Input: part model. Units: mm. Frame: model coordinates. Give positions to 0.01 mm unless a question says otherwise; leave off trailing zeros. Loops run counter-clockwise (first coordinate to the right, second up) from the corner with the lowest first, then second, coordinate; pieces in that order, holes last. Notation, with made-up numbers: M 75,32 L 115,32 A17 ccw 115,60 Z; hole C 34,80.5 d3. An arc over 180 degrees is marked long. Answer as a JSON object with one key per item and string values. Group by question number.
1) Section query A-A on z = 1. Return loops of the section in (x, y).
2) Section query B-B on x = -102. Return loops of the section in (y, z) (3 decimals), plus the area to 3 significant figures.
3) First-contact query: P1, Ø1.9, axis at y = 2.5, z = 37.5, coming from the -X side; P2, Ø1.9, axis at x = -59, y = 4, coming from the +Z side (3 decimals); P3, Ø1.9, axis at y = 2.5, z = 39.5, coming from the +X side; P4, Ø1.5, axis at x = -86, z = 26.5, coming from the -Y side. Flat tips, straight axial feed; report the tip coordinate or a pass-through.
4) Ray query, L1, parallel to X at y = 4.5, z = 29; L2, parallel to Z at x = 55, y = 1.5 (3 decimals); L3, parallel to X at y = 1.75, z = 1.5. Return the intervals inside material, ascending.
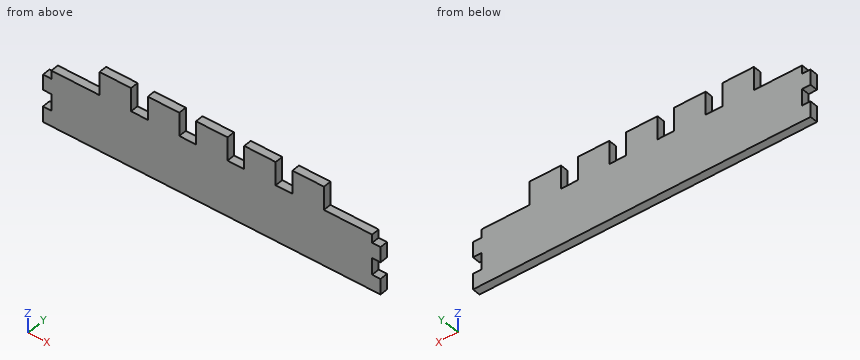
from build123d import *

# Parameters (mm, degrees)
SKETCH1_W           = 266.7
SKETCH1_H           = 57.15
BOSS_EXTRUDE1_DEPTH = 6.35
SKETCH3_W           = 24.892
SKETCH3_H           = 18.542
BOSS_EXTRUDE2_DEPTH = 6.35
SKETCH4_W           = 13.208
SKETCH4_H           = 13.208
CUT_EXTRUDE2_DEPTH  = 142.5717369
SKETCH5_W           = 295.464136086
SKETCH5_H           = 12.7
CUT_EXTRUDE3_DEPTH  = 142.5717369
SKETCH6_W           = 266.7
SKETCH6_H           = 12.446
BOSS_EXTRUDE3_DEPTH = 6.35


with BuildPart() as part:
    # Sketch1 → Boss-Extrude1 (new body)
    with BuildSketch(Plane(origin=(0, 0, 0), x_dir=(1, 0, 0), z_dir=(0, 1, 0))):
        Rectangle(SKETCH1_W, SKETCH1_H)
    extrude(amount=BOSS_EXTRUDE1_DEPTH)

    # Sketch3 → Boss-Extrude2 (add)
    with BuildSketch(Plane(origin=(0, 0, 0), x_dir=(1, 0, 0), z_dir=(0, 1, 0))):
        with Locations((-76.2, -37.846)):
            Rectangle(SKETCH3_W, SKETCH3_H)
        with Locations((-38.1, -37.846)):
            Rectangle(SKETCH3_W, SKETCH3_H)
        with Locations((0, -37.846)):
            Rectangle(SKETCH3_W, SKETCH3_H)
        with Locations((38.1, -37.846)):
            Rectangle(SKETCH3_W, SKETCH3_H)
        with Locations((76.2, -37.846)):
            Rectangle(SKETCH3_W, SKETCH3_H)
    extrude(amount=BOSS_EXTRUDE2_DEPTH)

    # Sketch4 → Cut-Extrude2 (cut, through all)
    with BuildSketch(Plane(origin=(0, 0, 0), x_dir=(1, 0, 0), z_dir=(0, 1, 0))):
        with Locations((-133.35, 22.225)):
            Rectangle(SKETCH4_W, SKETCH4_H)
        with Locations((133.35, 22.225)):
            Rectangle(SKETCH4_W, SKETCH4_H)
        with Locations((-133.35, -3.175)):
            Rectangle(SKETCH4_W, SKETCH4_H)
        with Locations((-133.35, -28.575)):
            Rectangle(SKETCH4_W, SKETCH4_H)
        with Locations((133.35, -3.175)):
            Rectangle(SKETCH4_W, SKETCH4_H)
        with Locations((133.35, -28.575)):
            Rectangle(SKETCH4_W, SKETCH4_H)
    extrude(amount=CUT_EXTRUDE2_DEPTH, mode=Mode.SUBTRACT)

    # Sketch5 → Cut-Extrude3 (cut, through all)
    with BuildSketch(Plane(origin=(0, 6.35, 0), x_dir=(1, 0, 0), z_dir=(0, 1, 0))):
        with Locations((7.963252738, 22.225)):
            Rectangle(SKETCH5_W, SKETCH5_H)
    extrude(amount=-CUT_EXTRUDE3_DEPTH, mode=Mode.SUBTRACT)

    # Sketch6 → Boss-Extrude3 (add)
    with BuildSketch(Plane(origin=(0, 6.35, 0), x_dir=(1, 0, 0), z_dir=(0, 1, 0))):
        with Locations((0, 9.652)):
            Rectangle(SKETCH6_W, SKETCH6_H)
    extrude(amount=-BOSS_EXTRUDE3_DEPTH)


solid = part.part
Output:
{
 "1": {"outline": "M -126.75,0 L 126.75,0 L 126.75,6.35 L -126.75,6.35 Z"},
 "2": {"outline": "M 0,-15.875 L 6.35,-15.875 L 6.35,28.575 L 0,28.575 Z", "area": "282 mm^2"},
 "3": {"P1": "stops at x = -88.65", "P2": "stops at z = 28.575", "P3": "stops at x = 88.65", "P4": "stops at y = 0"},
 "4": {"L1": "x = -88.65 to -63.75, -50.55 to -25.65, -12.45 to 12.45, 25.65 to 50.55, 63.75 to 88.65", "L2": "z = -15.875 to 28.575", "L3": "x = -126.75 to 126.75"}
}
